Model file for the job. Use its own axes, mm. A direction names the side the tool comes from. Round coordinates to 2 decimals unless told otherwise and drop trailing zeros. Order: outer loops, then holes, each group sorted by start corner. A loop starts at its lowest first (then second) coordinate and runs counter-clockwise, first axis right, second up. Notation, with made-up numbers: (76.5, -24) - (94.5, -24) arc R29 cw to (94.5, 2) - close; hole circle Ø6 at (31.5, 29.5). An arc over 180 degrees is marked (long way). Use one line per item in the form item = value.
from build123d import *

# Parameters (mm, degrees)
SKETCH1_W           = 153
SKETCH1_H           = 20
BOSS_EXTRUDE1_DEPTH = 3
SKETCH2_W           = 3
SKETCH2_H           = 20
BOSS_EXTRUDE2_DEPTH = 17
SKETCH3_W           = 150
SKETCH3_H           = 3
BOSS_EXTRUDE3_DEPTH = 17
SKETCH4_R           = 1.6
SKETCH4_R_2         = 1.598435099
CUT_EXTRUDE1_DEPTH  = 10
SKETCH6_W           = 30
SKETCH6_H           = 17
BOSS_EXTRUDE4_DEPTH = 4
SKETCH7_R           = 2.1
CUT_EXTRUDE3_DEPTH  = 243.348358538
SKETCH8_R           = 4
CUT_EXTRUDE4_DEPTH  = 2.5
SKETCH9_W           = 30
SKETCH9_H           = 17
BOSS_EXTRUDE5_DEPTH = 4
SKETCH12_R          = 2.1
CUT_EXTRUDE7_DEPTH  = 243.348358538
SKETCH13_R          = 4
CUT_EXTRUDE8_DEPTH  = 2.5
SKETCH14_W          = 30
SKETCH14_H          = 7
CUT_EXTRUDE9_DEPTH  = 3
CHAMFER8_SIZE       = 1
CHAMFER9_SIZE       = 3
SKETCH15_W          = 3.1
SKETCH15_H          = 17
CUT_EXTRUDE10_DEPTH = 3
SKETCH16_R          = 1.65
CUT_EXTRUDE11_DEPTH = 3
SKETCH17_R          = 3
CUT_EXTRUDE12_DEPTH = 6


with BuildPart() as part:
    # Sketch1 → Boss-Extrude1 (new body)
    with BuildSketch(Plane.XY):
        with Locations((164.901588409, -32.175360178)):
            Rectangle(SKETCH1_W, SKETCH1_H)
    extrude(amount=BOSS_EXTRUDE1_DEPTH)

    # Sketch2 → Boss-Extrude2 (add)
    with BuildSketch(Plane(origin=(0, 0, 0), x_dir=(-1, 0, 0), z_dir=(0, 0, -1))):
        with Locations((-89.901588409, -32.175360178)):
            Rectangle(SKETCH2_W, SKETCH2_H)
    extrude(amount=BOSS_EXTRUDE2_DEPTH)

    # Sketch3 → Boss-Extrude3 (add)
    with BuildSketch(Plane(origin=(0, 0, 0), x_dir=(-1, 0, 0), z_dir=(0, 0, -1))):
        with Locations((-166.401588409, -40.675360178)):
            Rectangle(SKETCH3_W, SKETCH3_H)
    extrude(amount=BOSS_EXTRUDE3_DEPTH)

    # Sketch4 → Cut-Extrude1 (cut)
    with BuildSketch(Plane.ZY.offset(-88.401588409)):
        with Locations((-13, -27.175360178)):
            Circle(SKETCH4_R)
        with Locations((-4, -27.175360178)):
            Circle(SKETCH4_R)
        with Locations((-4, -35.175360178)):
            Circle(SKETCH4_R)
        with Locations((-13, -35.175360178)):
            Circle(SKETCH4_R_2)
    extrude(amount=-CUT_EXTRUDE1_DEPTH, mode=Mode.SUBTRACT)

    # Sketch6 → Boss-Extrude4 (add)
    with BuildSketch(Plane(origin=(0, -39.175360178, 0), x_dir=(1, 0, 0), z_dir=(0, 1, 0))):
        with Locations((226.401588409, 8.5)):
            Rectangle(SKETCH6_W, SKETCH6_H)
    extrude(amount=BOSS_EXTRUDE4_DEPTH)

    # Sketch7 → Cut-Extrude3 (cut, through all)
    with BuildSketch(Plane(origin=(0, -35.175360178, 0), x_dir=(1, 0, 0), z_dir=(0, 1, 0))):
        with Locations(Location((219.401588409, 8.5, 0), (0, 0, 270))):
            Circle(SKETCH7_R)
        with Locations(Location((233.401588409, 8.5, 0), (0, 0, 270))):
            Circle(SKETCH7_R)
    extrude(amount=-CUT_EXTRUDE3_DEPTH, mode=Mode.SUBTRACT)

    # Sketch8 → Cut-Extrude4 (cut)
    with BuildSketch(Plane.XZ.offset(42.175360178)):
        with Locations(Location((219.401588409, -8.5, 0), (0, 0, 270))):
            Circle(SKETCH8_R)
        with Locations(Location((233.401588409, -8.5, 0), (0, 0, 270))):
            Circle(SKETCH8_R)
    extrude(amount=-CUT_EXTRUDE4_DEPTH, mode=Mode.SUBTRACT)

    # Sketch9 → Boss-Extrude5 (add)
    with BuildSketch(Plane(origin=(0, -39.175360178, 0), x_dir=(1, 0, 0), z_dir=(0, 1, 0))):
        with Locations((156.401588409, 8.5)):
            Rectangle(SKETCH9_W, SKETCH9_H)
    extrude(amount=BOSS_EXTRUDE5_DEPTH)

    # Sketch12 → Cut-Extrude7 (cut, through all)
    with BuildSketch(Plane(origin=(0, -35.175360178, 0), x_dir=(1, 0, 0), z_dir=(0, 1, 0))):
        with Locations(Location((163.401588409, 8.5, 0), (0, 0, 270))):
            Circle(SKETCH12_R)
        with Locations(Location((149.401588409, 8.5, 0), (0, 0, 270))):
            Circle(SKETCH12_R)
    extrude(amount=-CUT_EXTRUDE7_DEPTH, mode=Mode.SUBTRACT)

    # Sketch13 → Cut-Extrude8 (cut)
    with BuildSketch(Plane.XZ.offset(42.175360178)):
        with Locations(Location((163.401588409, -8.5, 0), (0, 0, 270))):
            Circle(SKETCH13_R)
        with Locations(Location((149.401588409, -8.5, 0), (0, 0, 270))):
            Circle(SKETCH13_R)
    extrude(amount=-CUT_EXTRUDE8_DEPTH, mode=Mode.SUBTRACT)

    # Sketch14 → Cut-Extrude9 (cut)
    with BuildSketch(Plane.XY.offset(3)):
        with Locations((221.401588409, -28.675360178)):
            Rectangle(SKETCH14_W, SKETCH14_H)
    extrude(amount=-CUT_EXTRUDE9_DEPTH, mode=Mode.SUBTRACT)

    # Chamfer8
    chamfer8_edges = [part.edges().sort_by_distance(p)[0] for p in [
        (236.401588409, -28.675360178, 0),
        (221.401588409, -32.175360178, 0),
        (206.401588409, -28.675360178, 0),
        (221.401588409, -25.175360178, 0),
    ]]
    chamfer(chamfer8_edges, length=CHAMFER8_SIZE)

    # Chamfer9
    chamfer9_edges = [part.edges().sort_by_distance(p)[0] for p in [
        (116.401588409, -39.175360178, 0),
        (191.401588409, -39.175360178, 0),
    ]]
    chamfer(chamfer9_edges, length=CHAMFER9_SIZE)

    # Sketch15 → Cut-Extrude10 (cut)
    with BuildSketch(Plane(origin=(0, -39.175360178, 0), x_dir=(1, 0, 0), z_dir=(0, 1, 0))):
        with Locations((209.851588409, 8.5)):
            Rectangle(SKETCH15_W, SKETCH15_H)
        with Locations((172.951588409, 8.5)):
            Rectangle(SKETCH15_W, SKETCH15_H)
        with Locations((139.851588409, 8.5)):
            Rectangle(SKETCH15_W, SKETCH15_H)
    extrude(amount=CUT_EXTRUDE10_DEPTH, mode=Mode.SUBTRACT)

    # Sketch16 → Cut-Extrude11 (cut)
    with BuildSketch(Plane(origin=(0, 0, 0), x_dir=(-1, 0, 0), z_dir=(0, 0, -1))):
        with Locations((-191.401588409, -27.175360178)):
            Circle(SKETCH16_R)
        with Locations(Location((-191.401588409, -35.175360178, 0), (0, 0, 322.694799034))):
            Circle(SKETCH16_R)
    extrude(amount=-CUT_EXTRUDE11_DEPTH, mode=Mode.SUBTRACT)

    # Sketch17 → Cut-Extrude12 (cut)
    with BuildSketch(Plane(origin=(0, 0, 0), x_dir=(-1, 0, 0), z_dir=(0, 0, -1))):
        with Locations((-191.401588409, -35.175360178)):
            Circle(SKETCH17_R)
    extrude(amount=CUT_EXTRUDE12_DEPTH, mode=Mode.SUBTRACT)


solid = part.part
(1) Slice it at A-A on z = -8.5. Count the separate pieces of the cut face and the enclosed holes in it, then the cut area to 3 significant figures.
Report:
separate_pieces = 5
enclosed_holes = 0
area = 594 mm2
(2) Tool access for faces 4 (the face through (174.502, -38, -1)), 5 (the face through (156, -35.175, -9)), 6 (the face through (89.88, -33.59, -4.21)), 7 (the face through (145.497, -40.943, -7.633)): list every direction of +Z, -Z, +X, -X, +Y, -Y with a clear straight run to the whole face (end or side of a thin tool).
Report:
face_4 = -Z, +Y
face_5 = -Z, +X, +Y
face_6 = -X
face_7 = -Y
(3) Pin check, flat tips, straight feed: pin 1 (2.5 mm diameter, centred on x = 191.4, y = -35.18, fed in from -Z); pin 2 (12 mm diameter, centred on x = 213, z = -8, fed in from +Y); pin 3 (6 mm diameter, centred on x = 204, y = -32.5, fed in from -Z); pin 4 (10 mm diameter, centred on y = -25.5, z = -6.5, fed in from +X). Stop position of each tip, or through.
Report:
pin_1 = through
pin_2 = -35.18
pin_3 = 0
pin_4 = 91.4
(4) Pull direction X, two halves, no side cores. Call faces 1 (the face through (147.352, -37.394, -8.955)), 2 (the face through (165, -38, -17)), 3 (the face through (241.402, -37, -5)): released by +X, released by -X, zero draft, split by the parting line, or undercut.
Report:
face_1 = undercut
face_2 = zero draft
face_3 = released by +X
(5) Slice it at B-B on x = 179. Give the cut face in (y, z).
Report:
outline = (-42.18, -17) - (-39.18, -17) - (-39.18, -3) - (-36.18, 0) - (-22.18, 0) - (-22.18, 3) - (-42.18, 3) - close
(6) Probe probe 1 along Y at (x, z) = (89.8, -13); probe 2 along X at (y, z) = (-35.75, -14.75); probe 3 along X at (y, z) = (-40.75, -7.5). List the from-to ranges inside material, lowest first. Write a range as [from, to].
Report:
probe_1 = [-42.18, -36.77], [-33.58, -28.78], [-25.58, -22.18]
probe_2 = [88.4, 91.4], [141.4, 171.4], [211.4, 241.4]
probe_3 = [88.4, 145.53], [153.27, 159.53], [167.27, 215.53], [223.27, 229.53], [237.27, 241.4]
